from build123d import *

# Parameters (mm, degrees)
ESQUISSE1_R                                        = 17.5
BOSS_EXTRU_1_DEPTH                                 = 10
CHAMBRAGE_POUR_VIS_T_TE_HEXAGONALE_M31_D           = 3.4
CHAMBRAGE_POUR_VIS_T_TE_HEXAGONALE_M31_CBORE_D     = 6.5
CHAMBRAGE_POUR_VIS_T_TE_HEXAGONALE_M31_CBORE_DEPTH = 3.4


with BuildPart() as part:
    # Esquisse1 → Boss.-Extru.1 (new body)
    with BuildSketch(Plane.XY):
        with BuildLine():
            Line((30, -5), (30, 5))
            Line((30, 5), (21.937410968, 5))
            ThreePointArc((21.937410968, 5), (0, 22.5), (-21.937410968, 5))
            Line((-21.937410968, 5), (-30, 5))
            Line((-30, 5), (-30, -5))
            Line((-30, -5), (-21.937410968, -5))
            ThreePointArc((-21.937410968, -5), (-17.781671131, -13.786303775), (-10.307764064, -20))
            Line((-10.307764064, -20), (-21.937410968, -31.33))
            Line((-21.937410968, -31.33), (21.345837795, -31.33))
            Line((21.345837795, -31.33), (10.307764064, -20))
            ThreePointArc((10.307764064, -20), (17.781671131, -13.786303775), (21.937410968, -5))
            Line((21.937410968, -5), (30, -5))
        make_face()
        Circle(ESQUISSE1_R, mode=Mode.SUBTRACT)
    extrude(amount=BOSS_EXTRU_1_DEPTH)

    # Chambrage pour vis à tête hexagonale M31 (through all)
    with Locations(Plane(origin=(25.97, 5, 5), x_dir=(1, 0, 0), z_dir=(0, 1, 0))):
        with Locations((0, 0)):
            chambrage_pour_vis_t_te_hexagonale_m31 = CounterBoreHole(CHAMBRAGE_POUR_VIS_T_TE_HEXAGONALE_M31_D / 2, CHAMBRAGE_POUR_VIS_T_TE_HEXAGONALE_M31_CBORE_D / 2, CHAMBRAGE_POUR_VIS_T_TE_HEXAGONALE_M31_CBORE_DEPTH)

    # Symétrie2: Chambrage pour vis à tête hexagonale M31 across plane
    add(chambrage_pour_vis_t_te_hexagonale_m31.mirror(Plane(origin=(0, 0, 0), x_dir=(0, 0, 1), z_dir=(1, 0, 0))), mode=Mode.SUBTRACT)


solid = part.part
Could you check a few things on this model? Use its own coordinates, in mm. A direction names the side the tool comes from. Coordinates: 2 decimals unless noted, no trailing zeros. Order: outer loops, then holes, each group sorted by start corner. A loop starts at its lowest first (then second) coordinate and runs counter-clockwise, first axis right, second up. Notation, with made-up numbers: (9, 6) -> (19, 6) arc R27 ccw to (19, 27) -> close; hole circle Ø2 at (55, 57). An arc over 180 degrees is marked (long way). One line per question, with ' | ' between items.
Q1. Thinking about a two-plate mould opening in X: for faces 4 (the face through (30, 0, 5)), 5 (the face through (-28, -5, 5)), 6 (the face through (-13.887, -10.648, 4.93)), which applies, pulls with the +X half, pulls with the -X half, needs draft (parallel to the pull), parting line crosses it, or undercut?
Return value:
face 4: pulls with the +X half | face 5: needs draft | face 6: undercut
Q2. Imagine slicing it at A-A on y = 0. Please give me the cut outline in (x, z), and give its area (3 significant figures).
Return value:
outline: (-30, 0) -> (-17.5, 0) -> (-17.5, 10) -> (-30, 10) -> close; (17.5, 0) -> (30, 0) -> (30, 10) -> (17.5, 10) -> close; hole circle Ø3.4 at (-25.97, 5); hole circle Ø3.4 at (25.97, 5) | area: 232 mm²
Q3. Imagine slicing it at D-D on y = -11. Please give me the cut outline in (x, z).
Return value:
outline: (-19.63, 0) -> (-13.61, 0) -> (-13.61, 10) -> (-19.63, 10) -> close; (13.61, 0) -> (19.63, 0) -> (19.63, 10) -> (13.61, 10) -> close
Q4. Imagine slicing it at B-B on z = 5. State how many separate pieces and enclosed holes the cut face has, and give its area (3 significant figures).
Return value:
separate pieces: 3 | enclosed holes: 1 | area: 1,020 mm²
Q5. Imagine slicing it at C-C on x = -25.97. Please give me the cut outline in (y, z).
Return value:
outline: (-5, 0) -> (5, 0) -> (5, 1.75) -> (1.6, 1.75) -> (1.6, 3.3) -> (-5, 3.3) -> close; (-5, 6.7) -> (1.6, 6.7) -> (1.6, 8.25) -> (5, 8.25) -> (5, 10) -> (-5, 10) -> close
Q6. If I drill on L1, parallel to X at y = -0.25, z = 5; L2, parallel to Y at x = 15, z = 6; L3, parallel to Z at x = -25.97, y = -0.5, over which ranges is the centre line in solid material (lowest first)?
Return value:
L1: -30 to -27.67, -24.27 to -17.5, 17.5 to 24.27, 27.67 to 30 | L2: -31.33 to -24.82, -16.77 to -9.01, 9.01 to 16.77 | L3: 0 to 3.3, 6.7 to 10
Q7. On a 3-axis mill with a long thin cutter (end or side, diameter ignored), from which of +Z, -Z, +X, -X, +Y, -Y can I reach the whole of each face in a straight line? I mean faces 1 (the face through (-25.9, 5, 1.6)), 2 (the face through (22.723, 3.324, 4.857)), 3 (the face through (26, 5, 1.6)). Say none if no direction works.
Return value:
face 1: +Z, -Z, -X, +Y | face 2: +Y | face 3: +Z, -Z, +X, +Y
Q8. I'm going to push flat-ended pins straight in: P1, Ø3, axis at x = 16.5, y = -4, coming from the +Z side; P2, Ø3, axis at y = 12, z = 6, coming from the +X side; P3, Ø5, axis at x = -27, z = 6, coming from the +Y side; P4, Ø5.5, axis at x = 25.97, z = 5, coming from the -Y side. Where does each tip first touch, or does it pass through?
Return value:
P1: z = 10 | P2: x = 19.9 | P3: y = 5 | P4: y = -5
